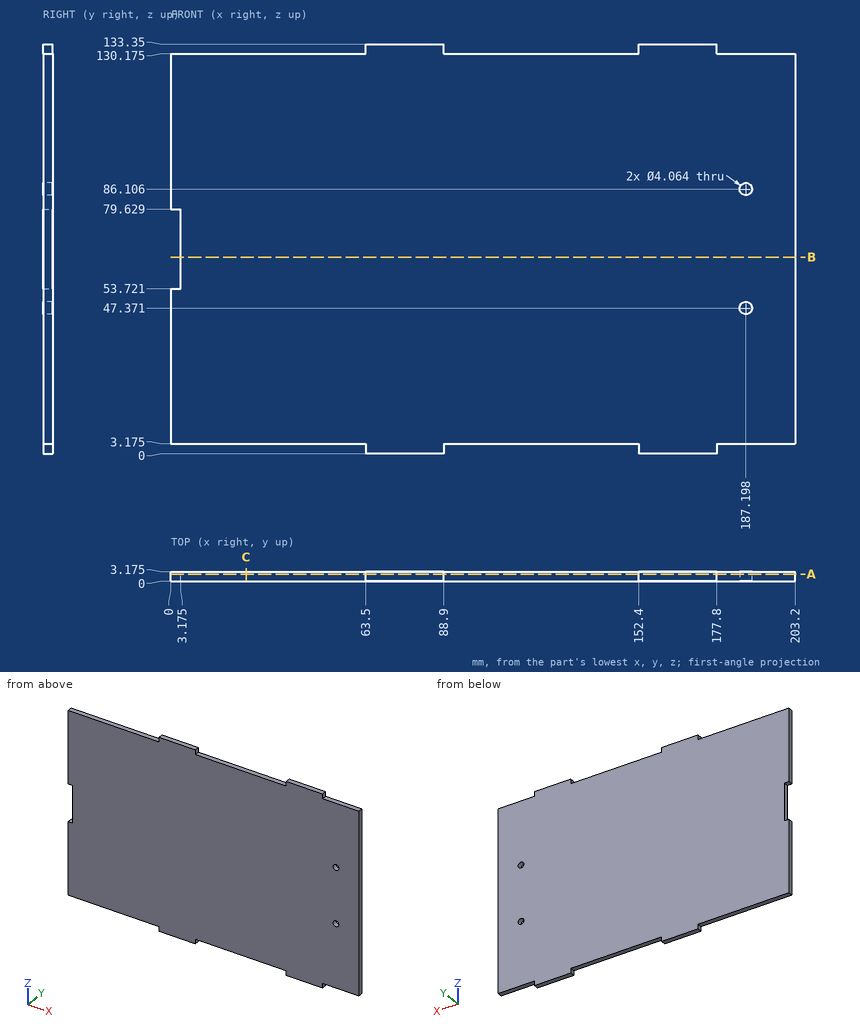
Here's the drawing with two shaded views (mm, measured from the low corner). I have some questions. Give positions to 0.01 mm unless a question says otherwise; leave off trailing zeros. Write each loop counter-clockwise with the first axis right and the second up, starting at its lowest first coordinate (ties: lowest second). Pieces come first, ordered by that corner, then holes. Notation, with made-up numbers: (87.5, 83.25) -> (113.5, 83.25) arc R10 cw to (113.5, 95.25) -> close; hole circle Ø3 at (87, 5). An arc over 180 degrees is marked (long way). Use one line per item in the form item = value.
1) If I drill on L1, parallel to X at y = 0.4, z = 47; L2, parallel to X at y = 2.75, z = 67 (3 decimals); L3, parallel to Z at x = 129, y = 1.5 (3 decimals), over which ranges is the centre line in solid material (lowest first)? Write a range as [from, to].
Verdict:
L1 = [0, 185.2], [189.2, 203.2]
L2 = [3.175, 203.2]
L3 = [3.175, 130.175]
2) Suppose I cut it at C-C (x = 24.5). Please give me the cut outline in (y, z) (3 decimals), and give its area (3 significant figures).
Verdict:
outline = (0, 3.175) -> (3.175, 3.175) -> (3.175, 130.175) -> (0, 130.175) -> close
area = 403 mm2
3) I'm going to push flat-ended pins straight in: pin 1 (1 mm diameter, centred on y = 0.5, z = 50.5, fed in from -X); pin 2 (1.6 mm diameter, centred on y = 2, z = 131.5, fed in from +X); pin 3 (1 mm diameter, centred on y = 2, z = 2, fed in from -X); pin 4 (1.6 mm diameter, centred on x = 194.5, y = 1, fed in from -Z) (3 decimals). Where does each tip first touch, or does it pass through?
Verdict:
pin_1 = 0
pin_2 = 177.8
pin_3 = 63.5
pin_4 = 3.175
4) Suppose I cut it at B-B (z = 64). Please give me the cut outline in (x, y) (3 decimals).
Verdict:
outline = (3.175, 0) -> (203.2, 0) -> (203.2, 3.175) -> (3.175, 3.175) -> close
5) Suppose I cut it at A-A (y = 2.4). Please give me the cut outline in (x, z) (3 decimals), and give its area (3 significant figures).
Verdict:
outline = (0, 3.175) -> (63.5, 3.175) -> (63.5, 0) -> (88.9, 0) -> (88.9, 3.175) -> (152.4, 3.175) -> (152.4, 0) -> (177.8, 0) -> (177.8, 3.175) -> (203.2, 3.175) -> (203.2, 130.175) -> (177.8, 130.175) -> (177.8, 133.35) -> (152.4, 133.35) -> (152.4, 130.175) -> (88.9, 130.175) -> (88.9, 133.35) -> (63.5, 133.35) -> (63.5, 130.175) -> (0, 130.175) -> (0, 79.629) -> (3.175, 79.629) -> (3.175, 53.721) -> (0, 53.721) -> close; hole circle Ø4.064 at (187.198, 47.371); hole circle Ø4.064 at (187.198, 86.106)
area = 26,000 mm2
